from build123d import *

# Parameters (mm, degrees)
F0_R     = 1.8629584398
F1_DEPTH = 9
F2_DEPTH = 10
F3_DEPTH = 1.1


with BuildPart() as f1:
    # F0 (on Top) → F1 (new body)
    with BuildSketch(Plane.XY):
        Polygon((18.5987912118, 38.7409813702), (10.9778223559, 38.7409813702), (8.437499404, 45.4549640417), (-1.9052419811, 45.4549640417), (-5.7157264091, 38.7409813702), (-8.618952008, 29.1236611083), (-11.5221776068, 19.5063408464), (-13.6186698187, 16.7213371643), (-14.8627730185, 15.0686565711), (-20.7560974635, 7.2398985219), (-23.6794371158, 3.3565014601), (-39.6471805871, 1.7233715625), (-49.2641143501, 11.3406926394), (-45.2721789479, 25.3130253404), (-57.0665337145, 21.3209297508), (-63.0544349551, 11.3406926394), (-55.4334707558, -7.5310315005), (-36.0181480646, -15.8781390637), (-8.9818555862, -7.5310315005), (-8.9818555862, -1.3614293421), (-4.0826620534, 6.2598437071), (5.7157254778, 6.2598437071), (5.7157254778, -5.8979014866), (12.2479852289, 1.7233715625), (12.2479852289, 17.6917538047), (16.7028524828, 14.5414304721), (18.3491399307, 10.9743302194), (21.5020161122, 12.4294450507), (19.3245969713, 17.1473771334), (14.606856741, 19.5063408464), (14.606856741, 28.7607442588), (22.4092733115, 28.7607442588), (22.4092733115, 36.1032277718), align=None)
        with Locations((6.0786283575, 42.0072451234)):
            Circle(F0_R, mode=Mode.SUBTRACT)
    extrude(amount=F1_DEPTH)

    # F0 (on Top) → F2 (join)
    with BuildSketch(Plane.XY):
        Polygon((18.5987912118, 38.7409813702), (10.9778223559, 38.7409813702), (8.437499404, 45.4549640417), (-1.9052419811, 45.4549640417), (-5.7157264091, 38.7409813702), (-8.618952008, 29.1236611083), (-11.5221776068, 19.5063408464), (-13.6186698187, 16.7213371643), (-14.8627730185, 15.0686565711), (-20.7560974635, 7.2398985219), (-23.6794371158, 3.3565014601), (-39.6471805871, 1.7233715625), (-49.2641143501, 11.3406926394), (-45.2721789479, 25.3130253404), (-57.0665337145, 21.3209297508), (-63.0544349551, 11.3406926394), (-55.4334707558, -7.5310315005), (-36.0181480646, -15.8781390637), (-8.9818555862, -7.5310315005), (-8.9818555862, -1.3614293421), (-4.0826620534, 6.2598437071), (5.7157254778, 6.2598437071), (5.7157254778, -5.8979014866), (12.2479852289, 1.7233715625), (12.2479852289, 17.6917538047), (16.7028524828, 14.5414304721), (18.3491399307, 10.9743302194), (21.5020161122, 12.4294450507), (19.3245969713, 17.1473771334), (14.606856741, 19.5063408464), (14.606856741, 28.7607442588), (22.4092733115, 28.7607442588), (22.4092733115, 36.1032277718), align=None)
        with Locations((6.0786283575, 42.0072451234)):
            Circle(F0_R, mode=Mode.SUBTRACT)
        Polygon((-8.618952008, 29.1236611083), (-5.7157264091, 38.7409813702), (-18.0544368923, 35.6552451849), (-16.0939348651, 34.2981147375), align=None)
        Polygon((-19.0954450518, 29.1236611083), (-8.618952008, 29.1236611083), (-16.0939348651, 34.2981147375), align=None)
        Polygon((-11.5221776068, 19.5063408464), (-8.618952008, 29.1236611083), (-19.0954450518, 29.1236611083), (-21.6834675521, 29.1236611083), (-18.9082012561, 24.8557609363), (-13.6186698187, 16.7213371643), align=None)
        Polygon((-19.0954450518, 29.1236611083), (-16.0939348651, 34.2981147375), (-23.8949824125, 35.0367799401), align=None)
        Polygon((-14.8627730185, 15.0686565711), (-13.6186698187, 16.7213371643), (-18.9082012561, 24.8557609363), (-20.3540053018, 16.6024911018), align=None)
        Polygon((-20.7560974635, 7.2398985219), (-14.8627730185, 15.0686565711), (-20.3540053018, 16.6024911018), (-22.9536294937, 17.3286292702), align=None)
        Polygon((-20.3540053018, 16.6024911018), (-18.9082012561, 24.8557609363), (-26.3009262924, 26.9207285705), align=None)
        Polygon((5.7157254778, -12.2489631176), (5.7157254778, -5.8979014866), (5.7157254778, 6.2598437071), (-4.0826620534, 6.2598437071), (-8.9818555862, -1.3614293421), (-8.9818555862, -7.5310315005), (0, -18.7814813107), (12.2479852289, -18.7814813107), (12.2479852289, -14.4264688715), align=None)
    extrude(amount=F2_DEPTH)

    # F3 (add): a face of the model
    f3_faces = [f1.faces().sort_by_distance(p)[0] for p in [
        (-14.7622843494, 10.8873438604, 10),
    ]]
    extrude(f3_faces, amount=-F3_DEPTH)


solid = f1.part
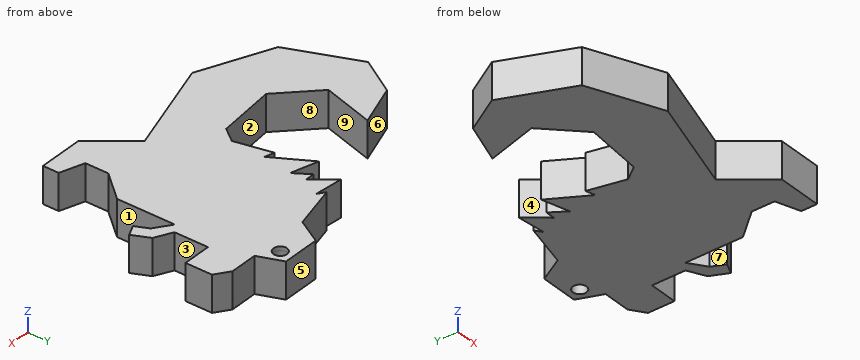
Model file for the job. Use its own axes, mm. Face numbers are marked on the shaded views. A direction names the side the tool comes from. Give positions to 0.01 mm unless a question says otherwise; leave off trailing zeros. Loops run counter-clockwise (first coordinate to the right, second up) from the corner with the lowest first, then second, coordinate; pieces in that order, holes last. Notation, with made-up numbers: (78, 59.5) -> (112, 59.5) arc R15 ccw to (112, 73.5) -> close; hole circle Ø9 at (55.25, 5.5). An arc over 180 degrees is marked (long way). Use a Markdown table: item, result. Add a question column.
(1) Mould opens along Y. For the marked faces 6, 7, 8 and 9 say: +Y half, -Y half, draft (parallel to the pull), parting line (faces both ways), or undercut.
(2) Slice it at A-A on y = 9.5. List the corners of the cut face in (x, z).
(3) Slice it at C-C on y = -3. List the corners of the cut face in (x, z).
(4) Slice it at B-B on x = -46.5. List the corners of the cut face in (y, z).
(5) Wall check: line 1 along X through (y, z) = (5.5, 2); line 2 along X through (y, z) = (19, 0.5); line 3 along Y through (x, z) = (-25, 6.5). Give the ranges that are in metal, low to high.
(6) Tool access for the marked faces 1, 2, 3, 4 and 5: list every direction of +Z, -Z, +X, -X, +Y, -Y with a clear straight run to the whole face (end or side of a thin tool).
(7) Drop flat-ended pins along their axis: pin 1 Ø2 at (x, y) = (6.08, 42.01) entering from +Z; pin 2 Ø3 at (x, z) = (-20.5, 2.5) entering from +Y; pin 3 Ø4 at (y, z) = (-5, 4.5) entering from +X; pin 4 Ø1 at (y, z) = (8, 2) entering from +X. Give the stop position or say it passes through.
Filled sheet:
| question | item | result |
|---|---|---|
| 1 | face 6 | +Y half |
| 1 | face 7 | -Y half |
| 1 | face 8 | undercut |
| 1 | face 9 | undercut |
| 2 | outline | (-62.31, 0) -> (-47.42, 0) -> (-47.42, 10) -> (-62.31, 10) -> close; (-21.25, 0) -> (12.25, 0) -> (12.25, 10) -> (-21.25, 10) -> close |
| 3 | outline | (-57.26, 0) -> (8.2, 0) -> (8.2, 10) -> (-57.26, 10) -> close |
| 4 | outline | (-11.37, 0) -> (8.58, 0) -> (8.58, 10) -> (-11.37, 10) -> close; (21.02, 0) -> (24.9, 0) -> (24.9, 10) -> (21.02, 10) -> close |
| 5 | line 1 | -60.7 to -43.42, -22.07 to 12.25 |
| 5 | line 2 | -58.46 to -47.08, -21.74 to 15.62 |
| 5 | line 3 | -12.48 to 3.22, 24.66 to 26.56 |
| 6 | face 1 | +Z, -Z, -Y |
| 6 | face 2 | +Z, -Z |
| 6 | face 3 | +Z, -Z, +X |
| 6 | face 4 | +Z, -Z, -X |
| 6 | face 5 | +Z, -Z, +X, -X, +Y |
| 7 | pin 1 | through |
| 7 | pin 2 | y = 34.86 |
| 7 | pin 3 | x = 8.2 |
| 7 | pin 4 | x = 12.25 |
